Autodesk Inventor part; units mm, degrees
sketch "Sketch1" plane through (0, 0, 0) normal (0, 0, 1) x (1, 0, 0)
  line L0 (0, 2.8582) -> (0, -2.8582) construction
  line L1 (-5.7775, 0) -> (5.7775, 0) construction
  line L2 (-48, -75) -> (48, -75)
  line L3 (48, -75) -> (48, 75)
  line L4 (48, 75) -> (-48, 75)
  line L5 (-48, 75) -> (-48, -75)
  line L6 (-48, -75) -> (48, 75) construction
  line L7 (48, -75) -> (-48, 75) construction
  point P0 (0, 0)
  point P1 (0, 0)
  dimension "d0" = 96
  dimension "d1" = 150
extrude "Extrusion1" add sketch "Sketch1" along normal blind 5
sketch "Sketch2" plane through (0, 0, 5) normal (0, 0, 1) x (1, 0, 0)
  line L0 (-48, 75) -> (-48, -75)
  line L1 (-48, 0) -> (-48, -15)
  line L2 (-48, -15) -> (-48, 15)
  line L3 (-48, 15) -> (-48, 45)
  line L4 (-48, 45) -> (-48, 75)
  line L5 (-48, -15) -> (-48, -45)
  line L6 (-48, -45) -> (-48, -75)
  line L7 (-48, -15) -> (-43, -15)
  line L8 (-43, -15) -> (-43, 15)
  line L9 (-43, 15) -> (-48, 15)
  line L10 (-48, 15) -> (-48, -15)
  line L11 (48, 75) -> (-48, 75)
  line L12 (-48, 45) -> (-43, 45)
  line L13 (-43, 45) -> (-43, 75)
  line L14 (-43, 75) -> (-48, 75)
  line L15 (-48, 75) -> (-48, 45)
  line L16 (-48, -45) -> (-43, -45)
  line L17 (-43, -45) -> (-43, -75)
  line L18 (-43, -75) -> (-48, -75)
  line L19 (-48, -75) -> (-48, -45)
  line L20 (-48, -75) -> (-33, -75)
  line L21 (-33, -75) -> (-33, -67)
  line L22 (-33, -67) -> (-48, -67)
  line L23 (-48, -67) -> (-48, -75)
  line L24 (-33, -75) -> (-3, -75)
  line L25 (-48, -75) -> (48, -75)
  line L26 (-3, -75) -> (27, -75)
  line L27 (-3, -75) -> (48, -75)
  line L28 (48, -75) -> (48, -67)
  line L29 (48, -67) -> (-3, -67)
  line L30 (-3, -67) -> (-3, -75)
  line L31 (-48, 75) -> (-33, 75)
  line L32 (-33, 75) -> (-33, 70)
  line L33 (-33, 70) -> (-48, 70)
  line L34 (-48, 70) -> (-48, 75)
  line L35 (48, -75) -> (48, 75)
  line L36 (-3, 75) -> (48, 75)
  line L37 (48, 75) -> (48, 70)
  line L38 (48, 70) -> (-3, 70)
  line L39 (-3, 70) -> (-3, 75)
  line L40 (-48, -75) -> (-33, -75)
  line L41 (-33, -75) -> (-33, -70)
  line L42 (-33, -70) -> (-48, -70)
  line L43 (-48, -70) -> (-48, -75)
  line L44 (-3, -75) -> (48, -75)
  line L45 (48, -75) -> (48, -70)
  line L46 (48, -70) -> (-3, -70)
  line L47 (-3, -70) -> (-3, -75)
  point P0 (0, 0)
  point P1 (-43, 70)
  point P2 (-33, 75)
  point P3 (-43, -67)
  point P4 (-43, -70)
  dimension "d4" = 15
  dimension "d5" = 30
  dimension "d6" = 30
  dimension "d7" = 30
  dimension "d8" = 30
  dimension "d9" = 5
  dimension "d10" = 15
  dimension "d12" = 30
  dimension "d13" = 30
  dimension "d14" = 51
  dimension "d15" = 5
  dimension "d18" = 15
  dimension "d23" = 8
  dimension "d24" = 5
extrude "Extrusion2" cut sketch "Sketch2" against normal blind 8 contours L11 L13 L33 L0 | L33 L13 L12 L0 | L11 L32 L33 L13 | L9 L8 L7 L0 | L11 L35 L38 L39 | L16 L17 L22 L0 | L22 L17 L42 L0 | L28 L25 L30 L46 | L42 L17 L18 L0 | L42 L21 L20 L17
sketch "Sketch4" plane through (0, 0, 5) normal (0, 0, 1) x (1, 0, 0)
  line L0 (-43, 15) -> (-43, -15)
  line L1 (-43, 0) -> (-18, 0)
  line L2 (-18, 0) -> (-18, -12.8)
  line L3 (-18, -12.8) -> (2.5, -12.8)
  line L4 (2.5, -12.8) -> (2.5, -10.2)
  line L5 (2.5, -10.2) -> (-18, -10.2)
  line L6 (-18, 0) -> (-18, 12.8)
  line L7 (-18, 12.8) -> (2.5, 12.8)
  line L8 (2.5, 12.8) -> (2.5, 10.2)
  line L9 (2.5, 10.2) -> (-18, 10.2)
  circle A0 centre (-3, -22.8) radius 3
  circle A1 centre (-3, 22.8) radius 3
  point P0 (0, 0)
  dimension "d25" = 25
  dimension "d26" = 12.8
  dimension "d27" = 20.5
  dimension "d28" = 2.6
  dimension "d29" = 12.8
  dimension "d30" = 20.5
  dimension "d31" = 2.6
  dimension "d36" = 6
  dimension "d37" = 6
  dimension "d39" = 15
  dimension "d40" = 10
  dimension "d41" = 15
  dimension "d42" = 10
extrude "Extrusion4" cut sketch "Sketch4" against normal blind 10
properties part number "Plaat voor" material "S235"
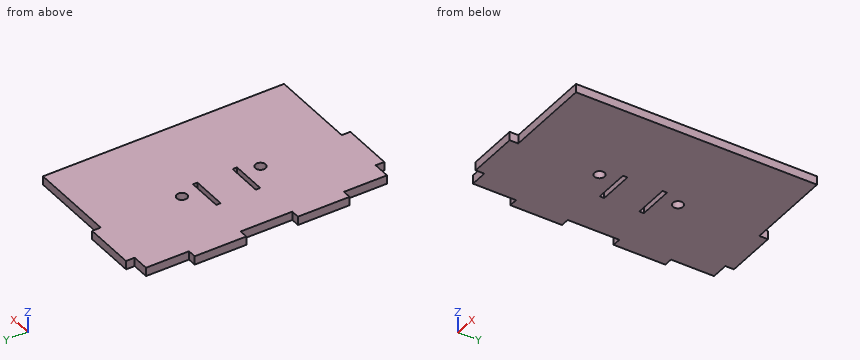
Input: part model. Units: mm. Frame: model coordinates. Give positions to 0.01 mm unless a question says otherwise; leave off trailing zeros. Order: outer loops, then holes, each group sorted by start corner. A loop starts at its lowest first (then second) coordinate and runs counter-clockwise, first axis right, second up.
1. Section B-B on z = 3.35. Give the number of separate pieces and of enclosed holes in the cut face, and give its area (3 significant figures).
Derived:
separate pieces: 1
enclosed holes: 4
area: 13,200 mm2
2. Section A-A on x = -12.5. Return the cut outline in (y, z).
Derived:
outline: (-75, 0) - (-12.8, 0) - (-12.8, 5) - (-75, 5) - close; (-10.2, 0) - (10.2, 0) - (10.2, 5) - (-10.2, 5) - close; (12.8, 0) - (75, 0) - (75, 5) - (12.8, 5) - close
3. Section C-C on y = 22.8. Return the cut outline in (x, z), and give its area (3 significant figures).
Derived:
outline: (-48, 0) - (-6, 0) - (-6, 5) - (-48, 5) - close; (0, 0) - (48, 0) - (48, 5) - (0, 5) - close
area: 450 mm2
4. Material intervals for L1, parallel to Y at x = -4, z = 2.2; L2, parallel to X at y = -14, z = 3.35; L3, parallel to X at y = 11.5, z = 1.75, sorted ascending.
Derived:
L1: y = -75 to -25.63, -19.97 to -12.8, -10.2 to 10.2, 12.8 to 19.97, 25.63 to 75
L2: x = -43 to 48
L3: x = -43 to -18, 2.5 to 48
5. Pin query (flat end, axial travel): pin 1 (2.5 mm diameter, centred on y = -3, z = 3, fed in from -X); pin 2 (2.5 mm diameter, centred on x = -40, z = 3.5, fed in from +Y); pin 3 (2.5 mm diameter, centred on x = 31.5, z = 3, fed in from -Y). Return the tip coordinate at first contact, or that it passes through.
Derived:
pin 1: stops at x = -43
pin 2: stops at y = 70
pin 3: stops at y = -70
6. Section D-D on x = 30. Return the cut outline in (y, z), and give its area (3 significant figures).
Derived:
outline: (-70, 0) - (70, 0) - (70, 5) - (-70, 5) - close
area: 700 mm2
